from build123d import *

# Parameters (mm, degrees)
SKETCH2_R          = 2
CUT_EXTRUDE1_DEPTH = 11.024968828
SKETCH3_R          = 4.7
SKETCH3_R_2        = 3
CUT_EXTRUDE2_DEPTH = 0.25


with BuildPart() as part:
    # Sketch1 → Revolve1 (revolve)
    with BuildSketch(Plane.XY, mode=Mode.PRIVATE) as revolve1_sk:
        with BuildLine():
            Line((0, 2), (0, -2))
            Line((0, -2), (6.5, -2))
            Line((6.5, -2), (6.5, -1.2))
            ThreePointArc((6.5, -1.2), (5.3, 0), (6.5, 1.2))
            Line((6.5, 1.2), (6.5, 2))
            Line((6.5, 2), (0, 2))
        make_face()
    revolve(revolve1_sk.sketch.rotate(Axis((0, 2, 0), (0, -1, 0)), 90), axis=Axis((0, 2, 0), (0, -1, 0)))

    # Sketch2 → Cut-Extrude1 (cut, through all)
    with BuildSketch(Plane(origin=(0, 2, 0), x_dir=(1, 0, 0), z_dir=(0, 1, 0))):
        with Locations(Location((0, 0, 0), (0, 0, 270))):
            Circle(SKETCH2_R)
    extrude(amount=-CUT_EXTRUDE1_DEPTH, mode=Mode.SUBTRACT)

    # Sketch3 → Cut-Extrude2 (cut)
    with BuildSketch(Plane(origin=(0, 2, 0), x_dir=(1, 0, 0), z_dir=(0, 1, 0))):
        with Locations(Location((0, 0, 0), (0, 0, 270))):
            Circle(SKETCH3_R)
        with Locations(Location((0, 0, 0), (0, 0, 270))):
            Circle(SKETCH3_R_2, mode=Mode.SUBTRACT)
    cut_extrude2 = extrude(amount=-CUT_EXTRUDE2_DEPTH, mode=Mode.SUBTRACT)

    # Sketch4 → Cut-Revolve1 (revolve, cut)
    with BuildSketch(Plane.XY, mode=Mode.PRIVATE) as cut_revolve1_sk:
        Polygon((4.7, 1.75), (4.2, 1.75), (4.7, 1.55), align=None)
    cut_revolve1 = revolve(cut_revolve1_sk.sketch.rotate(Axis((0, 1.75, 0), (0, 1, 0)), 270), axis=Axis((0, 1.75, 0), (0, 1, 0)), mode=Mode.SUBTRACT)

    # Mirror1: Cut-Extrude2, Cut-Revolve1 across plane
    add(cut_extrude2.mirror(Plane.ZX), mode=Mode.SUBTRACT)
    add(cut_revolve1.mirror(Plane.ZX), mode=Mode.SUBTRACT)


solid = part.part
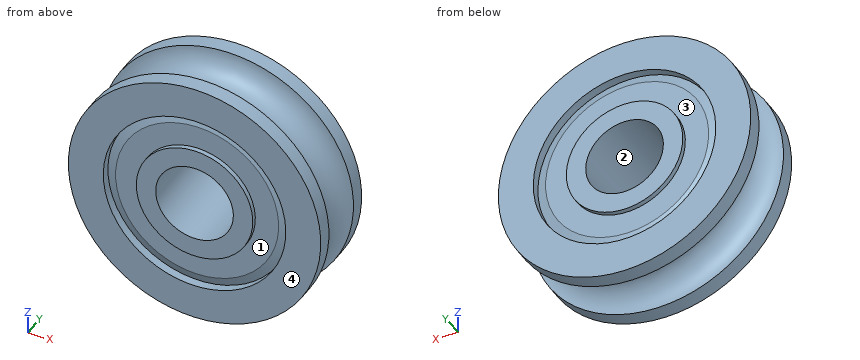
Work out the finished part from the listing and answer in its coordinate system (mm). Face numbers are marked on the shaded views. A direction names the side the tool comes from. Give positions to 0.01 mm unless a question says otherwise; leave off trailing zeros. Loops run counter-clockwise (first coordinate to the right, second up) from the corner with the lowest first, then second, coordinate; pieces in that order, holes last. Notation, with made-up numbers: M -20,67.5 L 27,67.5 A28 cw 27,102.5 Z; hole C -38.75,17.25 d4. An arc over 180 degrees is marked long. Use CSV: the item, a comma, the result in double quotes.
1) Which of the six approach directions +Z, -Z, +X, -X, +Y, -Y give full straight-line access (tool end or side, diameter ignored) to the marked faces 1 and 2?
Answer:
face 1,"-Y"
face 2,"+Y, -Y"
2) Consider L1, parallel to X at y = 1.9, z = 0; L2, parallel to Z at x = -1.25, y = -1.4; L3, parallel to Y at x = -5.5, z = 0. Determine where each line is inside the solid, lowest interval first.
Answer:
L1,"-6.5 to -4.7, -3 to -2, 2 to 3, 4.7 to 6.5"
L2,"-6.38 to -1.56, 1.56 to 6.38"
L3,"-2 to -0.66, 0.66 to 2"
3) Given P1, Ø2, axis at y = 1, z = 5, coming from the +X side; P2, Ø1, axis at y = 1.5, z = -2.5, coming from the +X side, each flat-ended and moving along its own axis, determine where each tip first touches the part or whether it passes through.
Answer:
P1,"x = 5.11"
P2,"x = 6.18"
4) Find section C-C on y = -0.7. Write down the section's boundary in (x, z).
Answer:
outline,"C 0,0 d11.05; hole C 0,0 d4"
5) Determine the mould class of the marked faces 3 and 4 for opening direction Z: released by +Z, released by -Z, zero draft, split by the parting line, or undercut.
Answer:
face 3,"undercut"
face 4,"zero draft"
